Read the model definition and answer for the solid it produces. Units are mm, in the model's axes. Face numbers are marked on the shaded views. Coordinates: 2 decimals unless noted, no trailing zeros. Write each loop counter-clockwise with the first axis right and the second up, starting at its lowest first coordinate (ties: lowest second). Pieces come first, ordered by that corner, then holes. Notation, with made-up numbers: (78.25, 1) -> (84.25, 1) arc R22 cw to (84.25, 31) -> close; hole circle Ø3 at (-21.75, 44.25). An arc over 180 degrees is marked (long way). Answer as a JSON object with one key per item and string values. Group by question number.
(1) Find section A-A (x = -31.5). Give the vertices of the cut face in (y, z) (3 decimals).
(2) Find section D-D (x = 37.5). Give the vertices of the cut face in (y, z) (3 decimals).
(3) Straight lines are drawn through the part: L1, parallel to Y at x = -15, z = 0.5; L2, parallel to Y at x = 11.43, z = -1.25; L3, parallel to Y at x = -29.5, z = 1. For each, find the intervals that lie inside material, in ascending order.
(4) Flat-ended cylindrical pins translate along their axes: P1, Ø7, axis at x = 11.43, y = -29.62, coming from the +Z side; P2, Ø1.5, axis at x = -37, z = 0, coming from the -Y side; P3, Ø1.5, axis at x = 0.5, z = -0.5, coming from the -Y side. Find the tip coordinate at first contact, or state that the pin passes through.
(5) Find section B-B (z = 1.5). Count the separate pieces of the cut face and the enclosed holes in it, then the cut area to 3 significant figures.
(6) Find section C-C (y = -9.5). Give the vertices of the cut face in (x, z) (3 decimals).
(7) For a pull along Y with two mould halves and no side action, classify the marked faces 1, 2, 3 and 4 as +Y half, -Y half, draft (parallel to the pull), parting line (faces both ways), or undercut.
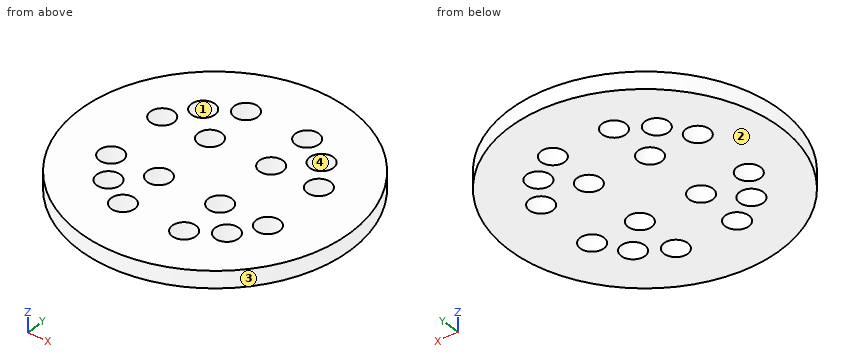
from build123d import *

# Parameters (mm, degrees)
F0_R     = 50.8
F0_R_2   = 4.445
F1_DEPTH = 3.175


with BuildPart() as f1:
    # F0 (on Top) → F1 (new body, symmetric)
    with BuildSketch(Plane.XY):
        Circle(F0_R)
        with Locations((-11.43, -29.621236)):
            Circle(F0_R_2, mode=Mode.SUBTRACT)
        with Locations((-29.279459, -12.279079)):
            Circle(F0_R_2, mode=Mode.SUBTRACT)
        with Locations((-22.124706, -22.77191)):
            Circle(F0_R_2, mode=Mode.SUBTRACT)
        with Locations((-11.43, -12.279079)):
            Circle(F0_R_2, mode=Mode.SUBTRACT)
        with Locations((11.43, -29.621236)):
            Circle(F0_R_2, mode=Mode.SUBTRACT)
        with Locations((22.124706, -22.77191)):
            Circle(F0_R_2, mode=Mode.SUBTRACT)
        with Locations((11.43, -12.279079)):
            Circle(F0_R_2, mode=Mode.SUBTRACT)
        with Locations((29.279459, -12.279079)):
            Circle(F0_R_2, mode=Mode.SUBTRACT)
        with Locations((-29.279459, 12.279079)):
            Circle(F0_R_2, mode=Mode.SUBTRACT)
        with Locations((-11.43, 12.279079)):
            Circle(F0_R_2, mode=Mode.SUBTRACT)
        with Locations((-22.124706, 22.77191)):
            Circle(F0_R_2, mode=Mode.SUBTRACT)
        with Locations((-11.43, 29.621236)):
            Circle(F0_R_2, mode=Mode.SUBTRACT)
        with Locations((11.43, 12.279079)):
            Circle(F0_R_2, mode=Mode.SUBTRACT)
        with Locations((22.124706, 22.77191)):
            Circle(F0_R_2, mode=Mode.SUBTRACT)
        with Locations((29.279459, 12.279079)):
            Circle(F0_R_2, mode=Mode.SUBTRACT)
        with Locations((11.43, 29.621236)):
            Circle(F0_R_2, mode=Mode.SUBTRACT)
    extrude(amount=F1_DEPTH, both=True)


solid = f1.part
Results below:
{
 "1": {"outline": "(-39.855, -3.175) -> (-16.13, -3.175) -> (-16.13, 3.175) -> (-39.855, 3.175) -> close; (-8.428, -3.175) -> (8.428, -3.175) -> (8.428, 3.175) -> (-8.428, 3.175) -> close; (16.13, -3.175) -> (39.855, -3.175) -> (39.855, 3.175) -> (16.13, 3.175) -> close"},
 "2": {"outline": "(-34.269, -3.175) -> (34.269, -3.175) -> (34.269, 3.175) -> (-34.269, 3.175) -> close"},
 "3": {"L1": "y = -48.53 to -32.27, -26.97 to -14.93, -9.63 to 9.63, 14.93 to 26.97, 32.27 to 48.53", "L2": "y = -49.5 to -34.07, -25.18 to -16.72, -7.83 to 7.83, 16.72 to 25.18, 34.07 to 49.5", "L3": "y = -41.36 to -16.72, -7.84 to 7.84, 16.72 to 41.36"},
 "4": {"P1": "passes through", "P2": "stops at y = -35.59", "P3": "stops at y = -50.8"},
 "5": {"separate pieces": "1", "enclosed holes": "16", "area": "7,110 mm2"},
 "6": {"outline": "(-49.904, -3.175) -> (-32.749, -3.175) -> (-32.749, 3.175) -> (-49.904, 3.175) -> close; (-25.81, -3.175) -> (-14.899, -3.175) -> (-14.899, 3.175) -> (-25.81, 3.175) -> close; (-7.961, -3.175) -> (7.961, -3.175) -> (7.961, 3.175) -> (-7.961, 3.175) -> close; (14.899, -3.175) -> (25.81, -3.175) -> (25.81, 3.175) -> (14.899, 3.175) -> close; (32.749, -3.175) -> (49.904, -3.175) -> (49.904, 3.175) -> (32.749, 3.175) -> close"},
 "7": {"face 1": "undercut", "face 2": "draft", "face 3": "parting line", "face 4": "undercut"}
}
